Here's how the part is built. I have some questions about the finished solid (model axes, mm). Give positions to 0.01 mm unless a question says otherwise; leave off trailing zeros. Write each loop counter-clockwise with the first axis right and the second up, starting at its lowest first coordinate (ties: lowest second). Pieces come first, ordered by that corner, then holes. Notation, with made-up numbers: (-24.75, -5) -> (23.25, -5) arc R25 cw to (23.25, 11) -> close; hole circle Ø7 at (-3.5, 5.5). An arc over 180 degrees is marked (long way). Answer as CSV lines item,"result". Start each with the question number.
from build123d import *

# Parameters (mm, degrees)
SKETCH1_R           = 78.35
SKETCH1_R_2         = 76.35
BOSS_EXTRUDE1_DEPTH = 1700
SKETCH5_R           = 15
CUT_EXTRUDE2_DEPTH  = 1704.607186237
SKETCH6_W           = 4.8
SKETCH6_H           = 270
CUT_EXTRUDE3_DEPTH  = 1704.607186346
CIRPATTERN1_COUNT   = 2
CIRPATTERN1_ANGLE   = 90


with BuildPart() as part:
    # Sketch1 → Boss-Extrude1 (new body)
    with BuildSketch(Plane.XY):
        Circle(SKETCH1_R)
        Circle(SKETCH1_R_2, mode=Mode.SUBTRACT)
    extrude(amount=BOSS_EXTRUDE1_DEPTH)

    # Sketch5 → Cut-Extrude2 (cut, through all)
    with BuildSketch(Plane(origin=(0, 0, 0), x_dir=(0, 0, -1), z_dir=(0.7071067811865489, -0.7071067811865462, 0))):
        with Locations(Location((-1034.89, 0, 0), (0, 0, 270))):
            Circle(SKETCH5_R)
    extrude(amount=CUT_EXTRUDE2_DEPTH, mode=Mode.SUBTRACT)

    # Sketch6 → Cut-Extrude3 (cut, symmetric)
    with BuildSketch(Plane(origin=(0, 0, 0), x_dir=(1, 0, 0), z_dir=(0, 1, 0))):
        with Locations((0, -150)):
            Rectangle(SKETCH6_W, SKETCH6_H)
    cut_extrude3 = extrude(amount=CUT_EXTRUDE3_DEPTH, both=True, mode=Mode.SUBTRACT)

    # CirPattern1: Cut-Extrude3 ×2 about axis
    cirpattern1_axis = Axis((0, 0, 0), (0, 0, 1))
    for i in range(1, CIRPATTERN1_COUNT):
        add(cut_extrude3.rotate(cirpattern1_axis, i * CIRPATTERN1_ANGLE / (CIRPATTERN1_COUNT - 1)), mode=Mode.SUBTRACT)


solid = part.part
Item 1: If we section it at A-A (y = 46): Please give me the cut outline in (x, z).
Item 2: If we section it at B-B (x = -24): Please give me the cut outline in (y, z), and give its area (3 significant figures).
Item 3: If I drill on line 1 (X direction, y = 0, z = 834); line 2 (X direction, y = -5.5, z = 470), over which ranges is the centre line in solid material (lowest first)? Write a range as [from, to].
Item 4: If we section it at C-C (z = 1099): Please give me the cut outline in (x, y).
Item 5: I'm going to push flat-ended pins straight in: pin 1 (6 mm diameter, centred on x = 15.5, z = 181, fed in from +Y); pin 2 (1 mm diameter, centred on y = -60.5, z = 1390, fed in from +X); pin 3 (1 mm diameter, centred on x = -7.5, z = 1122, fed in from -Y). Where does each tip first touch, or does it pass through?
Item 6: We'd pull the mould along Y, two halves only. Please class faces 1 (the face through (42.12, 66.065, 838.1)), 2 (the face through (17, -75, 1700)), 3 (the face through (-9.94, 75.7, 838.1)): released by +Y, released by -Y, zero draft, split by the parting line, or undercut.
Final values:
1,outline,"(-63.42, 0) -> (-60.94, 0) -> (-60.94, 1700) -> (-63.42, 1700) -> close; (60.94, 0) -> (63.42, 0) -> (63.42, 1700) -> (60.94, 1700) -> close"
2,outline,"(-74.58, 0) -> (-72.48, 0) -> (-72.48, 1700) -> (-74.58, 1700) -> close; (72.48, 0) -> (74.58, 0) -> (74.58, 1700) -> (72.48, 1700) -> close"
2,area,"7,150 mm2"
3,line 1,"[-78.35, -76.35], [76.35, 78.35]"
3,line 2,"[-78.16, -76.15], [76.15, 78.16]"
4,outline,"circle Ø156.7 at (0, 0); hole circle Ø152.7 at (0, 0)"
5,pin 1,"y = 77.35"
5,pin 2,"x = 50.39"
5,pin 3,"y = -78.04"
6,face 1,"split by the parting line"
6,face 2,"zero draft"
6,face 3,"undercut"
